Geometry: final body of the model. Coordinates: model frame, mm. Face numbers are marked on the shaded views. A direction names the side the tool comes from. Round coordinates to 2 decimals unless told otherwise and drop trailing zeros. Loops run counter-clockwise (first coordinate to the right, second up) from the corner with the lowest first, then second, coordinate; pieces in that order, holes last. Notation, with made-up numbers: M -1.5,74.25 L 34.5,74.25 A7 ccw 34.5,80.25 Z; hole C 22,-24 d7. An arc over 180 degrees is marked long. Answer as a JSON object with one key per item and string values.
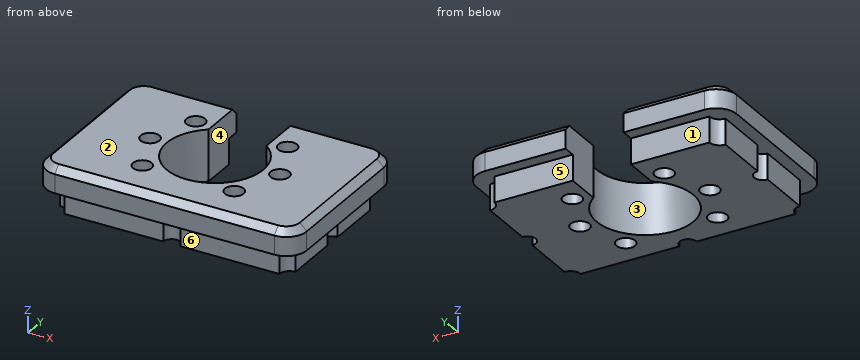
from build123d import *

# Parameters (mm, degrees)
SKETCH1_W           = 76.2
SKETCH1_H           = 50.8
BOSS_EXTRUDE1_DEPTH = 7.5
SKETCH2_W           = 68.85
SKETCH2_H           = 43.45
BOSS_EXTRUDE2_DEPTH = 7.5
SKETCH3_R           = 2.75
CUT_EXTRUDE1_DEPTH  = 49.184748624
FILLET1_R           = 6
SKETCH4_R           = 3
SKETCH4_R_2         = 2.5
CUT_EXTRUDE2_DEPTH  = 7.5
CHAMFER1_SIZE       = 2


with BuildPart() as part:
    # Sketch1 → Boss-Extrude1 (new body)
    with BuildSketch(Plane.XY):
        Rectangle(SKETCH1_W, SKETCH1_H)
    extrude(amount=-BOSS_EXTRUDE1_DEPTH)

    # Sketch2 → Boss-Extrude2 (add)
    with BuildSketch(Plane(origin=(0, 0, -7.5), x_dir=(-1, 0, 0), z_dir=(0, 0, -1))):
        Rectangle(SKETCH2_W, SKETCH2_H)
    extrude(amount=BOSS_EXTRUDE2_DEPTH)

    # Sketch3 → Cut-Extrude1 (cut, through all)
    with BuildSketch(Plane.XY):
        with Locations((-19, 0)):
            Circle(SKETCH3_R)
        with Locations((-13.435028843, 13.435028843)):
            Circle(SKETCH3_R)
        with Locations((13.435028843, 13.435028843)):
            Circle(SKETCH3_R)
        with Locations((19, 0)):
            Circle(SKETCH3_R)
        with Locations((13.435028843, -13.435028843)):
            Circle(SKETCH3_R)
        with Locations((-13.435028843, -13.435028843)):
            Circle(SKETCH3_R)
        with BuildLine():
            Line((8.5, 11.312493094), (8.5, 25.4))
            Line((8.5, 25.4), (-8.5, 25.4))
            Line((-8.5, 25.4), (-8.5, 11.312493094))
            ThreePointArc((-8.5, 11.312493094), (0, -14.15), (8.5, 11.312493094))
        make_face()
    extrude(amount=-CUT_EXTRUDE1_DEPTH, mode=Mode.SUBTRACT)

    # Fillet1
    fillet1_edges = [part.edges().sort_by_distance(p)[0] for p in [
        (-38.1, 25.4, -3.75),
        (38.1, 25.4, -3.75),
        (38.1, -25.4, -3.75),
        (-38.1, -25.4, -3.75),
    ]]
    fillet(fillet1_edges, radius=FILLET1_R)

    # Sketch4 → Cut-Extrude2 (cut)
    with BuildSketch(Plane(origin=(0, 0, -15), x_dir=(-1, 0, 0), z_dir=(0, 0, -1))):
        with Locations((-34.425, 21.725)):
            Circle(SKETCH4_R)
        with Locations((-34.425, -21.725)):
            Circle(SKETCH4_R)
        with Locations((-34.425, 0)):
            Circle(SKETCH4_R_2)
        with Locations((0, -21.725)):
            Circle(SKETCH4_R_2)
        with Locations((34.425, -21.725)):
            Circle(SKETCH4_R)
        with Locations((34.425, 0)):
            Circle(SKETCH4_R_2)
        with Locations((34.425, 21.725)):
            Circle(SKETCH4_R)
    extrude(amount=-CUT_EXTRUDE2_DEPTH, mode=Mode.SUBTRACT)

    # Chamfer1
    chamfer1_edges = [part.edges().sort_by_distance(p)[0] for p in [
        (-20.3, 25.4, 0),
        (0, -25.4, 0),
        (-38.1, 0, 0),
        (38.1, 0, 0),
        (20.3, 25.4, 0),
        (36.342640687, 23.642640687, 0),
        (-36.342640687, 23.642640687, 0),
        (-36.342640687, -23.642640687, 0),
        (36.342640687, -23.642640687, 0),
    ]]
    chamfer(chamfer1_edges, length=CHAMFER1_SIZE)


solid = part.part
1) Pull-direction query (Y, two-part tool) for the marked faces 1, 2 and 3; classes: +Y half, -Y half, draft (parallel to the pull), parting line (faces both ways), or undercut.
Results:
{"face 1": "+Y half", "face 2": "draft", "face 3": "undercut"}
2) Section query D-D (z = -10.25). Count the separate pieces of the cut face and the enclosed holes in it, and give its area (3 significant figures).
Results:
{"separate pieces": "1", "enclosed holes": "6", "area": "2,020 mm2"}
3) Pin query (flat end, axial travel): P1, Ø6, axis at y = -8.5, z = -11.5, coming from the +X side (3 decimals); P2, Ø4, axis at x = -17.5, z = -11.5, coming from the -Y side (3 decimals); P3, Ø4, axis at y = -11, z = -10.5, coming from the -X side (3 decimals). Return the tip coordinate at first contact, or that it passes through.
Results:
{"P1": "x = 34.425", "P2": "y = -21.725", "P3": "x = -34.425"}
4) Section query A-A (y = 0). Return the cut outline in (x, z) (3 decimals).
Results:
{"outline": "M -38.1,-7.5 L -31.925,-7.5 L -31.925,-15 L -21.75,-15 L -21.75,0 L -36.1,0 L -38.1,-2 Z; M -16.25,-15 L -14.15,-15 L -14.15,0 L -16.25,0 Z; M 14.15,-15 L 16.25,-15 L 16.25,0 L 14.15,0 Z; M 21.75,-15 L 31.925,-15 L 31.925,-7.5 L 38.1,-7.5 L 38.1,-2 L 36.1,0 L 21.75,0 Z"}
5) Section query C-C (x = 0). Return the cut outline in (y, z) (3 decimals).
Results:
{"outline": "M -25.4,-7.5 L -19.225,-7.5 L -19.225,-15 L -14.15,-15 L -14.15,0 L -23.4,0 L -25.4,-2 Z"}
6) Section query B-B (x = 19). Return the cut outline in (y, z) (3 decimals).
Results:
{"outline": "M -25.4,-7.5 L -21.725,-7.5 L -21.725,-15 L -2.75,-15 L -2.75,0 L -23.4,0 L -25.4,-2 Z; M 2.75,-15 L 21.725,-15 L 21.725,-7.5 L 25.4,-7.5 L 25.4,-2 L 23.4,0 L 2.75,0 Z"}
7) Ray query, line 1 (Y direction, x = -19, z = -11.25) (3 decimals); line 2 (Y direction, x = 0, z = -5.75); line 3 (X direction, y = 3, z = -2.5). Return the intervals inside material, ascending.
Results:
{"line 1": "-21.725 to -2.75, 2.75 to 21.725", "line 2": "-25.4 to -14.15", "line 3": "-38.1 to -13.83, 13.83 to 38.1"}
8) Reachability of the marked faces 4, 5 and 6 from +Z, -Z, +X, -X, +Y, -Y: full face, straight path, thin tool, end or side. Return the list, or none.
Results:
{"face 4": "+Z, -Z, +Y", "face 5": "-Z, +X, -X, +Y", "face 6": "-Z, +X, -X, -Y"}
